Geometry check sheet. Reference: drawing and pictorial views, mm from the part's lowest x, y, z. A direction names the side the tool comes from. Give positions to 0.01 mm unless a question says otherwise; leave off trailing zeros. Write each loop counter-clockwise with the first axis right and the second up, starting at its lowest first coordinate (ties: lowest second). Pieces come first, ordered by that corner, then holes.
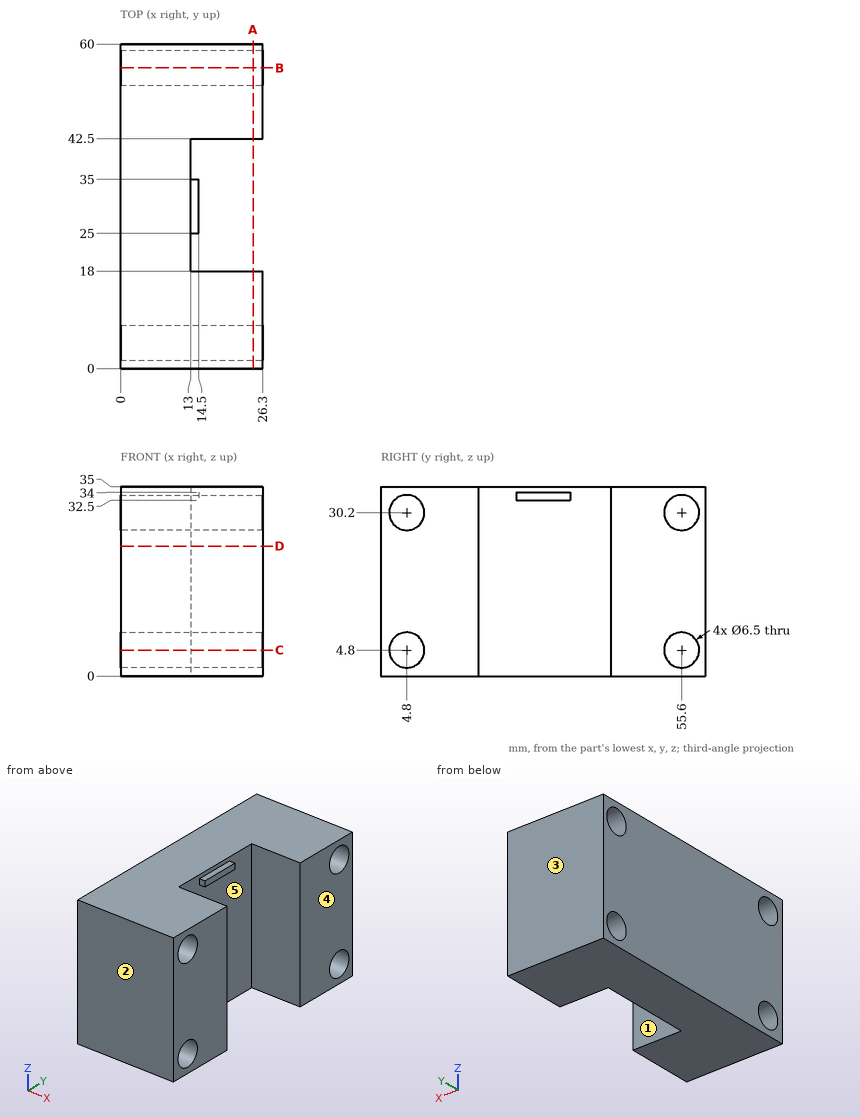
Item 1: Sectioned sample at B-B on y = 55.6. Record the cut outline in (x, z).
Answer key:
outline: (0, 0) - (26.3, 0) - (26.3, 1.55) - (0, 1.55) - close; (0, 8.05) - (26.3, 8.05) - (26.3, 26.95) - (0, 26.95) - close; (0, 33.45) - (26.3, 33.45) - (26.3, 35) - (0, 35) - close
Item 2: Sectioned sample at A-A on x = 24.5. Record the cut outline in (y, z).
Answer key:
outline: (0, 0) - (18, 0) - (18, 35) - (0, 35) - close; (42.5, 0) - (60, 0) - (60, 35) - (42.5, 35) - close; hole circle Ø6.5 at (4.8, 4.8); hole circle Ø6.5 at (4.8, 30.2); hole circle Ø6.5 at (55.6, 4.8); hole circle Ø6.5 at (55.6, 30.2)
Item 3: Set-up check for the marked faces 1 and 2: record each of +Z, -Z, +X, -X, +Y, -Y from which the full face is reachable in a straight line by a thin tool's end or side.
Answer key:
face 1: +Z, -Z, +X
face 2: +Z, -Z, +X, -X, -Y
Item 4: Sectioned sample at C-C on z = 4.8. Record the cut outline in (x, y), then the cut area to 3 significant figures.
Answer key:
outline: (0, 0) - (26.3, 0) - (26.3, 1.55) - (0, 1.55) - close; (0, 8.05) - (26.3, 8.05) - (26.3, 18) - (13, 18) - (13, 42.5) - (26.3, 42.5) - (26.3, 52.35) - (0, 52.35) - close; (0, 58.85) - (26.3, 58.85) - (26.3, 60) - (0, 60) - close
area: 910 mm2
Item 5: Scan lines: line 1 along Y through (x, z) = (16.5, 30.2); line 2 along Y through (x, z) = (23, 7); line 3 along Y through (x, z) = (5.5, 30.2). Record each from-to range of solid material in increasing order.
Answer key:
line 1: y = 0 to 1.55, 8.05 to 18, 42.5 to 52.35, 58.85 to 60
line 2: y = 0 to 2.41, 7.19 to 18, 42.5 to 53.21, 57.99 to 60
line 3: y = 0 to 1.55, 8.05 to 52.35, 58.85 to 60
Item 6: Sectioned sample at D-D on z = 24. Record the cut outline in (x, y), then the cut area to 3 significant figures.
Answer key:
outline: (0, 0) - (26.3, 0) - (26.3, 18) - (13, 18) - (13, 42.5) - (26.3, 42.5) - (26.3, 60) - (0, 60) - close
area: 1,250 mm2
Item 7: Depth check by flat-ended pin: pin 1 (1.2 mm diameter, centred on y = 30, z = 33, fed in from +X); pin 2 (0.8 mm diameter, centred on x = 13.5, y = 28, fed in from +Z); pin 3 (0.8 mm diameter, centred on x = 14, y = 32, fed in from -Z). Enter the tip coordinate at first touch or a pass-through.
Answer key:
pin 1: stops at x = 14.5
pin 2: stops at z = 34
pin 3: stops at z = 32.5
Item 8: Release check for a two-part mould opening along Y. For the marked faces 3, 4 and 5 record: released by +Y, released by -Y, zero draft, split by the parting line, or undercut.
Answer key:
face 3: released by +Y
face 4: zero draft
face 5: undercut
